Input: part model. Units: mm. Frame: model coordinates. A direction names the side the tool comes from. Coordinates: 2 decimals unless noted, no trailing zeros. Write each loop counter-clockwise with the first axis right and the second up, starting at its lowest first coordinate (ties: lowest second). Pieces come first, ordered by that corner, then holes. Notation, with made-up numbers: (86.25, -13) - (139.25, -13) arc R23 cw to (139.25, 19) - close; hole circle Ø8 at (78, 88.25). An arc over 180 degrees is marked (long way). Use a Markdown table: item, result. Add a question column.
Q1. Section query B-B (y = 63.5). Return the cut outline in (x, z), then the cut area to 3 significant figures.
Q2. Section query D-D (z = 192.5). Return the cut outline in (x, y), then the cut area to 3 significant figures.
Q3. Section query A-A (y = -15). Return the cut outline in (x, z), then the cut area to 3 significant figures.
Q4. Mould query, pull axis Z, two halves, no side actions, for faces 6 (the face through (12, 95.25, 125)), 7 (the face through (-56.972, -101.689, 125.381)), 8 (the face through (0, 63.4, 241.4)). Classes: released by +Z, released by -Z, zero draft, split by the parting line, or undercut.
Q5. Pin query (flat end, axial travel): P1, Ø14, axis at x = -13.5, z = 240.5, coming from the -Y side; P2, Ø6.5, axis at x = -10, z = 240, coming from the -Y side; P3, Ø11.5, axis at x = -50.8, y = 63.5, coming from the -Z side; P4, Ø4, axis at y = 9, z = 4, coming from the +X side. Return the tip coordinate at first contact, or that it passes through.
Q6. Set-up query: faces 1 (the face through (56.469, -67.847, 6.261)), 2 (the face through (-13, -57.912, 241)), 3 (the face through (26, -105, 234.95)), 4 (the face through (24, -1, 234.95)), 5 (the face through (24, 101.6, 241)). Return all of +Z, -Z, +X, -X, +Y, -Y with unobstructed straight access to the full face (end or side cutting, diameter ignored); none if empty.
Q7. Material intervals for probe 1 along Y at (x, z) = (-50, 4); probe 2 along X at (y, z) = (63, 7); probe 3 along Y at (x, z) = (23, 80.5), sorted ascending. Write a range as from..to.
Q8. Section query C-C (x = -50.8). Return the cut outline in (y, z).
from build123d import *

# Parameters (mm, degrees)
F0_W     = 139.7
F0_H     = 241.3
F1_DEPTH = 12.7
F3_D     = 14.2875
F5_W     = 139.7
F5_H     = 203.2
F6_DEPTH = 12.7
F8_DEPTH = 6.35


with BuildPart() as f1:
    # F0 (on Top) → F1 (new body)
    with BuildSketch(Plane.XY):
        Rectangle(F0_W, F0_H)
    extrude(amount=F1_DEPTH)

    # F3 (through all)
    with Locations(Plane.XY.offset(12.7)):
        with Locations((-50.8, 63.5), (50.8, 63.5), (50.8, -63.5), (-50.8, -63.5)):
            Hole(F3_D / 2)



with BuildPart() as f6:
    # F5 (on offset) → F6 (new body)
    with BuildSketch(Plane(origin=(0, 0, 247.65), x_dir=(1, 0, 0), z_dir=(0, 0, -1))):
        with Locations((25.4, 0)):
            Rectangle(F5_W, F5_H)
        with BuildLine():
            Line((-5.588, -69.088), (-19.812, -69.088))
            ThreePointArc((-19.812, -69.088), (-25.4, -63.5), (-19.812, -57.912))
            Line((-19.812, -57.912), (-5.588, -57.912))
            ThreePointArc((-5.588, -57.912), (0, -63.5), (-5.588, -69.088))
        make_face(mode=Mode.SUBTRACT)
        with BuildLine():
            ThreePointArc((56.388, -69.088), (50.8, -63.5), (56.388, -57.912))
            Line((56.388, -57.912), (70.612, -57.912))
            ThreePointArc((70.612, -57.912), (76.2, -63.5), (70.612, -69.088))
            Line((70.612, -69.088), (56.388, -69.088))
        make_face(mode=Mode.SUBTRACT)
        with BuildLine():
            Line((-5.588, 57.912), (-19.812, 57.912))
            ThreePointArc((-19.812, 57.912), (-25.4, 63.5), (-19.812, 69.088))
            Line((-19.812, 69.088), (-5.588, 69.088))
            ThreePointArc((-5.588, 69.088), (0, 63.5), (-5.588, 57.912))
        make_face(mode=Mode.SUBTRACT)
        with BuildLine():
            Line((56.388, 69.088), (70.612, 69.088))
            ThreePointArc((70.612, 69.088), (76.2, 63.5), (70.612, 57.912))
            Line((70.612, 57.912), (56.388, 57.912))
            ThreePointArc((56.388, 57.912), (50.8, 63.5), (56.388, 69.088))
        make_face(mode=Mode.SUBTRACT)
    extrude(amount=F6_DEPTH)


with BuildPart() as f1_1:
    add(f1.part)

    add(f6.part)  # F8 merges F6
    # F7 (on face) → F8 (join, symmetric)
    with BuildSketch(Plane.XZ.offset(101.6)):
        Polygon((95.25, 234.95), (-44.45, 234.95), (-69.85, 12.7), (69.85, 12.7), align=None)
    extrude(amount=F8_DEPTH, both=True)

    # F9: F1 across plane


with BuildPart() as f1_2:
    add(f1_1.part)
    add(f1_1.part.mirror(Plane.XZ))


solid = f1_2.part
Values follow:
| question | item | result |
|---|---|---|
| 1 | outline | (-69.85, 0) - (-57.94, 0) - (-57.94, 12.7) - (-69.85, 12.7) - close; (-44.45, 234.95) - (-25.4, 234.95) - (-25.4, 247.65) - (-44.45, 247.65) - close; (-43.66, 0) - (43.66, 0) - (43.66, 12.7) - (-43.66, 12.7) - close; (0, 234.95) - (50.8, 234.95) - (50.8, 247.65) - (0, 247.65) - close; (57.94, 0) - (69.85, 0) - (69.85, 12.7) - (57.94, 12.7) - close; (76.2, 234.95) - (95.25, 234.95) - (95.25, 247.65) - (76.2, 247.65) - close |
| 1 | area | 2,540 mm2 |
| 2 | outline | (-49.3, -107.95) - (90.4, -107.95) - (90.4, -95.25) - (-49.3, -95.25) - close; (-49.3, 95.25) - (90.4, 95.25) - (90.4, 107.95) - (-49.3, 107.95) - close |
| 2 | area | 3,550 mm2 |
| 3 | outline | (-69.85, 0) - (69.85, 0) - (69.85, 12.7) - (-69.85, 12.7) - close; (-44.45, 234.95) - (95.25, 234.95) - (95.25, 247.65) - (-44.45, 247.65) - close |
| 3 | area | 3,550 mm2 |
| 4 | face 6 | undercut |
| 4 | face 7 | released by +Z |
| 4 | face 8 | zero draft |
| 5 | P1 | y = -107.95 |
| 5 | P2 | y = -101.6 |
| 5 | P3 | through |
| 5 | P4 | x = 69.85 |
| 6 | face 1 | -Z |
| 6 | face 2 | +Z |
| 6 | face 3 | +Z, +X, -X, -Y |
| 6 | face 4 | +X, -X |
| 6 | face 5 | +Z, +X, -X, +Y |
| 7 | probe 1 | -120.65..-70.6, -56.4..56.4, 70.6..120.65 |
| 7 | probe 2 | -69.85..-57.93, -43.67..43.67, 57.93..69.85 |
| 7 | probe 3 | -107.95..-95.25, 95.25..107.95 |
| 8 | outline | (-120.65, 0) - (-70.64, 0) - (-70.64, 12.7) - (-95.25, 12.7) - (-95.25, 179.39) - (-107.95, 179.39) - (-107.95, 12.7) - (-120.65, 12.7) - close; (-56.36, 0) - (56.36, 0) - (56.36, 12.7) - (-56.36, 12.7) - close; (70.64, 0) - (120.65, 0) - (120.65, 12.7) - (107.95, 12.7) - (107.95, 179.39) - (95.25, 179.39) - (95.25, 12.7) - (70.64, 12.7) - close |
